The model under review builds one solid part; all positions refer to its coordinate system, in mm. Face numbers are marked on the shaded views. A direction names the side the tool comes from. Round coordinates to 2 decimals unless told otherwise and drop trailing zeros. Order: outer loops, then holes, each group sorted by start corner. A loop starts at its lowest first (then second) coordinate and runs counter-clockwise, first axis right, second up.
```python
from build123d import *

# Parameters (mm, degrees)
EXTRUDE_START         = -2
SKETCH_1_R            = 18
EXTRUDE_1_DEPTH       = 15
SKETCH_2_R            = 13.000000001
CUT_EXTRUDE_1_DEPTH   = 10.5
SKETCH_3_R            = 10.200000005
CUT_EXTRUDE_2_DEPTH   = 31.64670615
SKETCH_4_R            = 1.5
CUT_EXTRUDE_2_2_DEPTH = 31.64670615


with BuildPart() as part:
    # Эскиз1 → Вытянуть1 (new body)
    with BuildSketch(Plane(origin=(0, 0, 0), x_dir=(1, 0, 0), z_dir=(0, 1, 0)).offset(EXTRUDE_START)):
        with Locations(Location((0, -1.754002071, 0), (0, 0, 270))):
            Circle(SKETCH_1_R)
    extrude(amount=EXTRUDE_1_DEPTH)

    # Эскиз2 → Вырез-Вытянуть1 (cut)
    with BuildSketch(Plane.XZ.offset(2)):
        with Locations(Location((3.8e-08, 1.754001981, 0), (0, 0, 270))):
            Circle(SKETCH_2_R)
    extrude(amount=-CUT_EXTRUDE_1_DEPTH, mode=Mode.SUBTRACT)

    # Эскиз3 → Cut-Extrude 2 (cut, through all)
    with BuildSketch(Plane(origin=(0, 13, 0), x_dir=(1, 0, 0), z_dir=(0, 1, 0))):
        with Locations(Location((3.8e-08, -1.754001981, 0), (0, 0, 270))):
            Circle(SKETCH_3_R)
    extrude(amount=-CUT_EXTRUDE_2_DEPTH, mode=Mode.SUBTRACT)

    # Эскиз4 → Cut-Extrude 2 2 (cut, through all)
    with BuildSketch(Plane(origin=(0, 13, 0), x_dir=(1, 0, 0), z_dir=(0, 1, 0))):
        with Locations(Location((0, 13.791856832, 0), (0, 0, 270))):
            Circle(SKETCH_4_R)
        with Locations(Location((15.545858903, -1.754002071, 0), (0, 0, 270))):
            Circle(SKETCH_4_R)
        with Locations(Location((0, -17.299860974, 0), (0, 0, 270))):
            Circle(SKETCH_4_R)
        with Locations(Location((-15.545858903, -1.754002071, 0), (0, 0, 270))):
            Circle(SKETCH_4_R)
    extrude(amount=-CUT_EXTRUDE_2_2_DEPTH, mode=Mode.SUBTRACT)


solid = part.part
```
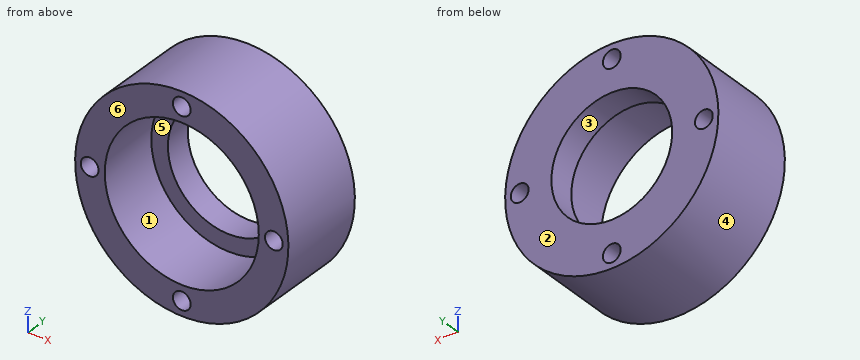
(1) Consider section D-D (y = 10.5). Write out the cut boundary in (x, z), and give its area (3 significant figures).
Data:
outline: circle Ø36 at (0, 1.75); hole circle Ø3 at (-15.55, 1.75); hole circle Ø20.4 at (0, 1.75); hole circle Ø3 at (0, -13.79); hole circle Ø3 at (0, 17.3); hole circle Ø3 at (15.55, 1.75)
area: 663 mm2
(2) Insertion check: pin 1 (3 mm diameter, centred on x = 8.5, y = 11, fed in from -Z); pin 2 (5 mm diameter, centred on x = 10.5, y = -0.5, fed in from +Z); pin 3 (3 mm diameter, centred on x = 3.5, z = -5, fed in from -Y); pin 4 (5 mm diameter, centred on x = 13.5, y = 11, fed in from -Z). Each pin has a flat end and moves straight along its axis. Give the tip position at first contact, or say it passes through.
Data:
pin 1: stops at z = -14.83
pin 2: stops at z = 17.88
pin 3: passes through
pin 4: stops at z = -12.49
(3) Consider section B-B (z = -14). Write out the cut boundary in (x, y).
Data:
outline: (-8.71, -2) - (-1.49, -2) - (-1.49, 13) - (-8.71, 13) - close; (1.49, -2) - (8.71, -2) - (8.71, 13) - (1.49, 13) - close
(4) Consider section A-A (x = 0). Write out the cut boundary in (y, z), and give its area (3 significant figures).
Data:
outline: (-2, -16.25) - (13, -16.25) - (13, -15.29) - (-2, -15.29) - close; (-2, -12.29) - (13, -12.29) - (13, -8.45) - (8.5, -8.45) - (8.5, -11.25) - (-2, -11.25) - close; (-2, 14.75) - (8.5, 14.75) - (8.5, 11.95) - (13, 11.95) - (13, 15.8) - (-2, 15.8) - close; (-2, 18.8) - (13, 18.8) - (13, 19.75) - (-2, 19.75) - close
area: 85.2 mm2
(5) To check wall thickness, follow probe 1 along X at (y, z) = (2.75, 2); probe 2 along Z at (x, y) = (-1, 7); probe 3 along X at (y, z) = (2.25, -8.5). State the ranges of each line that lie inside material, in increasing order.
Data:
probe 1: x = -18 to -17.03, -14.07 to -13, 13 to 14.07, 17.03 to 18
probe 2: z = -16.22 to -14.91, -12.67 to -11.21, 14.72 to 16.18, 18.42 to 19.73
probe 3: x = -14.79 to -7.99, 7.99 to 14.79
(6) Draft analysis for pull direction X (two halves, no side actions). For the marked faces 3, 4, 5 and 6, state which applies: pulls with the +X half, pulls with the -X half, needs draft (parallel to the pull), parting line crosses it, or undercut.
Data:
face 3: undercut
face 4: parting line crosses it
face 5: undercut
face 6: needs draft
(7) Consider section C-C (x = -4). Write out the cut boundary in (y, z).
Data:
outline: (-2, -15.8) - (13, -15.8) - (13, -7.63) - (8.5, -7.63) - (8.5, -10.62) - (-2, -10.62) - close; (-2, 14.12) - (8.5, 14.12) - (8.5, 11.14) - (13, 11.14) - (13, 19.3) - (-2, 19.3) - close
(8) For the marked faces 1 and 2, list the 3-axis set-ups (+Z, -Z, +X, -X, +Y, -Y) from which the entire face can be reached by the end or side of a thin tool; tool diameter is ignored.
Data:
face 1: -Y
face 2: +Z, -Z, +X, -X, +Y
